from build123d import *

# Parameters (mm, degrees)
CROSSRECESS_DEPTH = 0.825
DRAFT9_ANGLE      = 30
FILLET5_R         = 0.3
SKETCH10_W        = 0.5
SKETCH10_H        = 1.5


with BuildPart() as part:
    # Sketch1 → Base (revolve)
    with BuildSketch(Plane.XY):
        Polygon((50, 1.5), (2.65, 1.5), (1.65, 1.5), (0.55, 2.6), (0, 2.6), (0, 0), (50, 0), align=None)
    revolve(axis=Axis((4.515812911, 0, 0), (-1, 0, 0)))

    # Sketch6 → CrossRecess (cut)
    with BuildSketch(Plane(origin=(0, 0, 0), x_dir=(0, 0, -1), z_dir=(1, 0, 0))):
        Polygon((0.32, 0.32), (0.32, 1.6), (-0.32, 1.6), (-0.32, 0.32), (-1.6, 0.32), (-1.6, -0.32), (-0.32, -0.32), (-0.32, -1.6), (0.32, -1.6), (0.32, -0.32), (1.6, -0.32), (1.6, 0.32), align=None)
    extrude(amount=CROSSRECESS_DEPTH, mode=Mode.SUBTRACT)

    # Draft9
    draft9_faces = [part.faces().sort_by_distance(p)[0] for p in [
        (0.4125, -1.6, 0),
        (0.4125, 0, 1.6),
        (0.4125, 0, -1.6),
        (0.4125, 1.6, 0),
    ]]
    draft(draft9_faces, Plane(origin=(0, 2.6, 0), x_dir=(0, 0, -1), z_dir=(-1, 0, 0)), DRAFT9_ANGLE)

    # Fillet5
    fillet5_edges = [part.edges().sort_by_distance(p)[0] for p in [
        (0.4125, 0.32, 0.32),
        (0.4125, -0.32, 0.32),
        (0.4125, -0.32, -0.32),
        (0.4125, 0.32, -0.32),
    ]]
    fillet(fillet5_edges, radius=FILLET5_R)

    # Sketch10 → Revolve2 (revolve)
    with BuildSketch(Plane.XY):
        with Locations((1.9, 0.75)):
            Rectangle(SKETCH10_W, SKETCH10_H)
    revolve(axis=Axis((62.228915663, 0, 0), (-1, 0, 0)))


solid = part.part
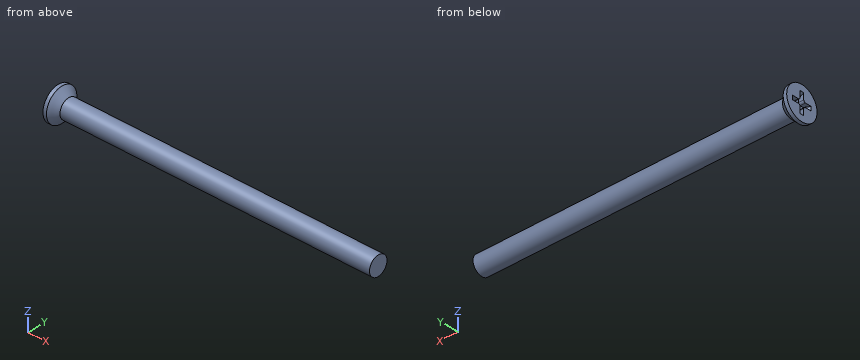
The model under review builds one solid part; all positions refer to its coordinate system, in mm. Round coordinates to 2 decimals unless told otherwise and drop trailing zeros. Order: outer loops, then holes, each group sorted by start corner. A loop starts at its lowest first (then second) coordinate and runs counter-clockwise, first axis right, second up. Notation, with made-up numbers: (-24.5, 60.5) -> (31.5, 60.5) arc R17 ccw to (31.5, 74.5) -> close; hole circle Ø10 at (-31.5, 3). An arc over 180 degrees is marked (long way). Use CSV: the item, a comma, the result in double quotes. Start each with the question number.
(1) Wall thickness on probe 1 along Y at (x, z) = (38, 0.1); probe 2 along Y at (x, z) = (9, -0.5); probe 3 along X at (y, z) = (2, -0.4): over which ranges is each line inside the solid? List them lowest first. Write a range as from..to.
(2) Consider section A-A on x = 3. Write out the cut boundary in (y, z).
(3) Insertion check: pin 1 (3 mm diameter, centred on x = 6.5, y = -1, fed in from -Z); pin 2 (0.7 mm diameter, centred on x = 0.5, z = -1, fed in from -Y); pin 3 (0.7 mm diameter, centred on x = 0.5, y = -1.5, fed in from -Z). Each pin has a flat end and moves straight along its axis. Give the tip position at first contact, or say it passes through.
Responses:
1,probe 1,"-1.5..1.5"
1,probe 2,"-1.41..1.41"
1,probe 3,"0..1.11"
2,outline,"circle Ø3 at (0, 0)"
3,pin 1,"z = -1.5"
3,pin 2,"y = -2.52"
3,pin 3,"z = -2.33"
